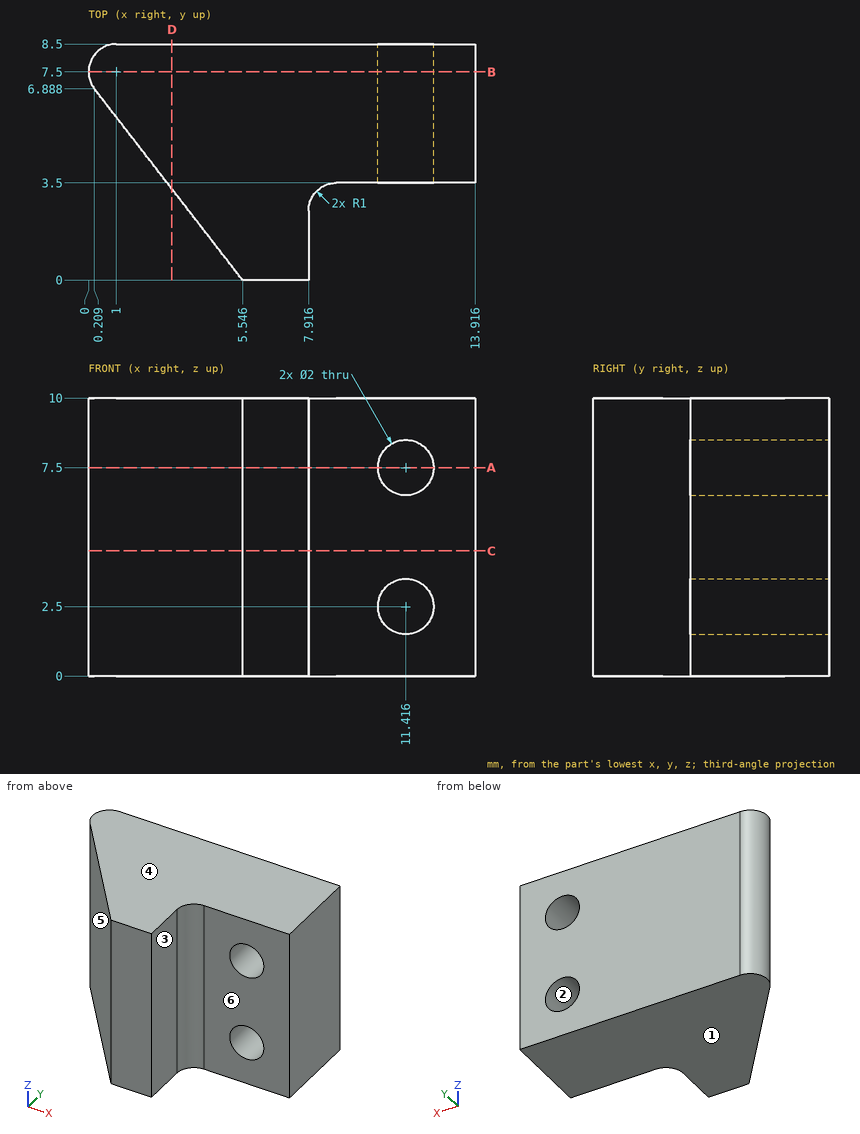
Could you check a few things on this drawing? It's one solid part, dimensions in mm from its lowest x, y, z. A direction names the side the tool comes from. Coordinates: 2 decimals unless noted, no trailing zeros. Write each loop counter-clockwise with the first axis right and the second up, starting at its lowest first coordinate (ties: lowest second). Pieces come first, ordered by that corner, then holes. Notation, with made-up numbers: M -31.5,-27.75 L 18.5,-27.75 A21 ccw 18.5,-2.75 Z; hole C -32,-32.5 d1. An arc over 180 degrees is marked long. Answer as CSV lines item,"result". Start each with the question number.
Q1. Suppose I cut it at A-A, the plane z = 7.5. List the corners of the cut face in (x, y) for me (1 decimal).
Q2. I need wall thicknesses on probe 1 along Y at (x, z) = (12.75, 7.5); probe 2 along X at (y, z) = (4.75, 1.75) (1 decimal); probe 3 along Y at (x, z) = (4.5, 8.5). Which ranges of each line are inside material? Lowest first, please. Write a range as [from, to].
Q3. Suppose I cut it at C-C, the plane z = 4.5. List the corners of the cut face in (x, y) for me (1 decimal).
Q4. Will these pins go through, and if not, where does the flat tip stop? pin 1 Ø4 at (x, z) = (11, 5.5) entering from -Y; pin 2 Ø1.8 at (x, z) = (11.42, 2.5) entering from -Y; pin 3 Ø1 at (x, z) = (3, 8.5) entering from -Y; pin 4 Ø1.5 at (y, z) = (1.5, 5.5) entering from -X.
Q5. If we mould it in two halves opening along Z, with no side actions, what happens to the marked faces 1, 2, 3 and 4? For each: pulls with the +Z half, pulls with the -Z half, needs draft (parallel to the pull), parting line crosses it, or undercut.
Q6. For the marked faces 5 and 6, which set-ups out of +Z, -Z, +X, -X, +Y, -Y let a thin tool reach every point of the face, with its end or its side?
Q7. Suppose I cut it at B-B, the plane y = 7.5. List the corners of the cut face in (x, z) for me, then the cut area to 3 significant figures.
Q8. Suppose I cut it at D-D, the plane x = 3. List the corners of the cut face in (y, z) for me (1 decimal).
Entries:
1,outline,"M 0.2,6.9 L 5.5,0 L 7.9,0 L 7.9,2.5 A1 cw 8.9,3.5 L 10.4,3.5 L 10.4,8.5 L 1,8.5 A1 ccw Z; M 12.4,3.5 L 13.9,3.5 L 13.9,8.5 L 12.4,8.5 Z"
2,probe 1,"y = [3.5, 8.5]"
2,probe 2,"x = [1.9, 10.8], [12.1, 13.9]"
2,probe 3,"y = [1.35, 8.5]"
3,outline,"M 0.2,6.9 L 5.5,0 L 7.9,0 L 7.9,2.5 A1 cw 8.9,3.5 L 13.9,3.5 L 13.9,8.5 L 1,8.5 A1 ccw Z"
4,pin 1,"stops at y = 3.5"
4,pin 2,"passes through"
4,pin 3,"stops at y = 2.64"
4,pin 4,"stops at x = 3.8"
5,face 1,"pulls with the -Z half"
5,face 2,"undercut"
5,face 3,"needs draft"
5,face 4,"pulls with the +Z half"
6,face 5,"+Z, -Z, -X, -Y"
6,face 6,"+Z, -Z, +X, -Y"
7,outline,"M 0,0 L 13.92,0 L 13.92,10 L 0,10 Z; hole C 11.42,2.5 d2; hole C 11.42,7.5 d2"
7,area,"133 mm²"
8,outline,"M 3.3,0 L 8.5,0 L 8.5,10 L 3.3,10 Z"
